Can you work these out from the model? Positions are in its coordinate system, mm. Face numbers are marked on the shaded views. A direction names the side the tool comes from. Give positions to 0.01 mm unless a question says otherwise; leave off trailing zeros. Write each loop counter-clockwise with the first axis right and the second up, starting at its lowest first coordinate (ties: lowest second). Pieces come first, ordered by that corner, then holes. Notation, with made-up numbers: M -27.5,56 L 7.5,56 A11 ccw 7.5,62 Z; hole C -25.5,81 d2. An arc over 180 degrees is marked long. Write each question's results on one line, items separated by ' | '.
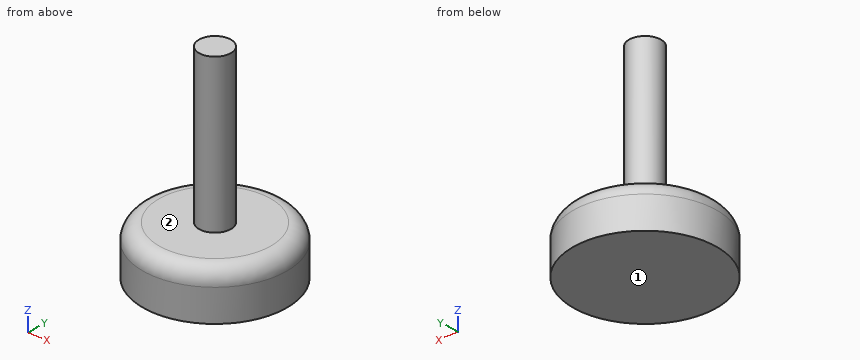
Autodesk Inventor part; units mm, degrees
ref_plane "YZ Plane" through (0, 0, 0) normal (1, 0, 0) x (0, 1, 0)
ref_plane "XZ Plane" through (0, 0, 0) normal (0, 1, 0) x (-1, 0, 0)
ref_plane "XY Plane" through (0, 0, 0) normal (0, 0, 1) x (1, 0, 0)
sketch "Sketch1" plane through (0, 0, 0) normal (0, 0, 1) x (1, 0, 0)
  circle A0 centre (0, 0) radius 14.2875
  dimension "d0" = 28.575
extrude "Extrusion1" add sketch "Sketch1" along normal blind 9.525
sketch "Sketch2" plane through (0, 0, 9.525) normal (0, 0, 1) x (1, 0, 0)
  circle A0 centre (0, 0) radius 14.2875
  circle A1 centre (0, 0) radius 3.175
  dimension "d3" = 6.35
extrude "Extrusion2" add sketch "Sketch2" along normal blind 30.48 contours A1
thread "Thread1"
fillet "Fillet1" radius 3.175 1 edges at (-14.2875, 0, 9.525)
properties part number "23015T81_leveling_feet"
Item 1: For the marked faces 1 and 2, which set-ups out of +Z, -Z, +X, -X, +Y, -Y let a thin tool reach every point of the face, with its end or its side?
Geometry says:
face 1: -Z, +X, -X, +Y, -Y | face 2: +Z
Item 2: I want a section at C-C, the plane z = 28.5. Please give me the cut outline in (x, y) (3 decimals).
Geometry says:
outline: C 0,0 d6.35
Item 3: I'm going to push flat-ended pins straight in: pin 1 (8 mm diameter, centred on x = 5.5, z = 21.5, fed in from -Y); pin 2 (8 mm diameter, centred on y = 0.5, z = 31, fed in from +X) (3 decimals); pin 3 (10 mm diameter, centred on y = 5, z = 17, fed in from -X) (3 decimals). Where does each tip first touch, or does it pass through?
Geometry says:
pin 1: stops at y = -2.8 | pin 2: stops at x = 3.175 | pin 3: stops at x = -3.175
Item 4: If I drill on line 1 (Z direction, x = -4.5, y = -4.75) (3 decimals); line 2 (Z direction, x = 8, y = 11.5); line 3 (X direction, y = -2.5, z = 6.5), over which ranges is the centre line in solid material (lowest first)? Write a range as from..to.
Geometry says:
line 1: z = 0..9.525 | line 2: z = 0..7.65 | line 3: x = -14.06..14.06
